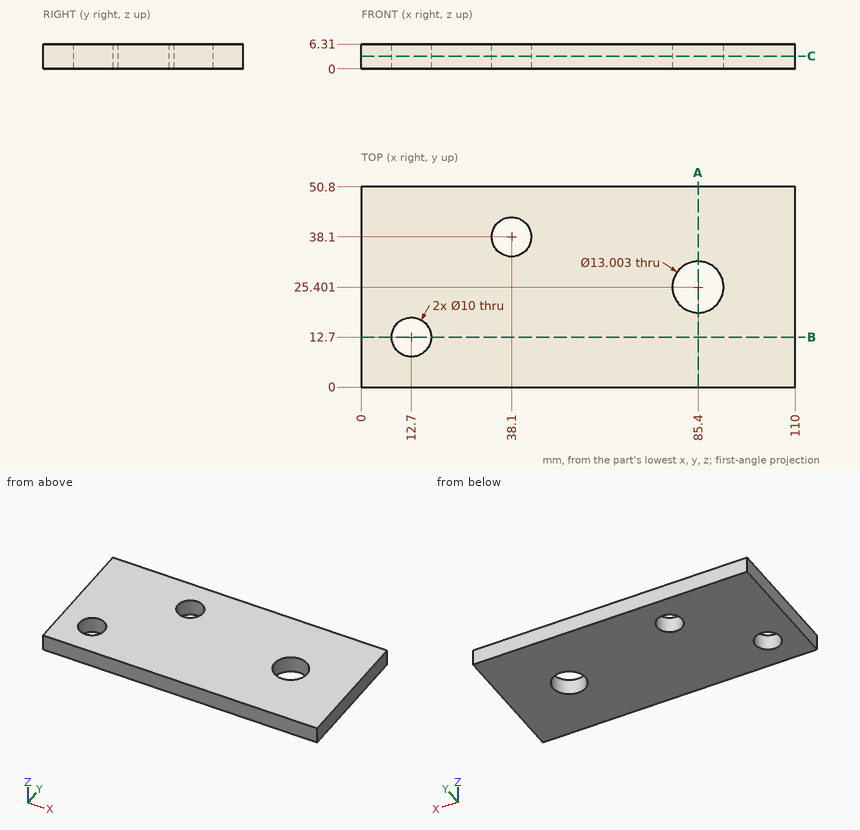
Verification items for this drawing (mm, ordinates from the low corner). Round coordinates to 2 decimals unless told otherwise and drop trailing zeros. Order: outer loops, then holes, each group sorted by start corner. A loop starts at its lowest first (then second) coordinate and runs counter-clockwise, first axis right, second up.
1) Cross-section at A-A, the plane x = 85.4. Record the cut outline in (y, z).
Geometry says:
outline: (0, 0) - (18.9, 0) - (18.9, 6.31) - (0, 6.31) - close; (31.9, 0) - (50.8, 0) - (50.8, 6.31) - (31.9, 6.31) - close
2) Cross-section at C-C, the plane z = 3.25. Record the cut outline in (x, y).
Geometry says:
outline: (0, 0) - (110, 0) - (110, 50.8) - (0, 50.8) - close; hole circle Ø10 at (12.7, 12.7); hole circle Ø10 at (38.1, 38.1); hole circle Ø13 at (85.4, 25.4)
3) Cross-section at B-B, the plane y = 12.7. Record the cut outline in (x, z), plus the area to 3 significant figures.
Geometry says:
outline: (0, 0) - (7.7, 0) - (7.7, 6.31) - (0, 6.31) - close; (17.7, 0) - (110, 0) - (110, 6.31) - (17.7, 6.31) - close
area: 631 mm2
4) Material ranges on line 1 (Y direction, x = 12.7, z = 4); line 2 (Y direction, x = 85.4, z = 3); line 3 (X direction, y = 20.5, z = 5), recorded low to high.
Geometry says:
line 1: y = 0 to 7.7, 17.7 to 50.8
line 2: y = 0 to 18.9, 31.9 to 50.8
line 3: x = 0 to 81.13, 89.67 to 110
